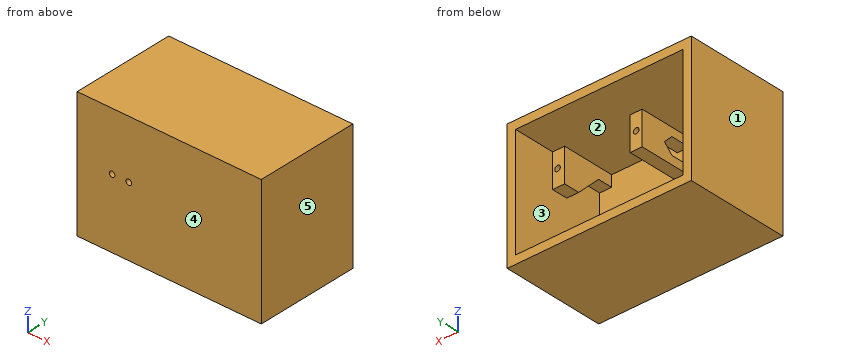
Autodesk Inventor part; units mm, degrees
ref_plane "YZ Plane" through (0, 0, 0) normal (1, 0, 0) x (0, 1, 0)
ref_plane "XZ Plane" through (0, 0, 0) normal (0, 1, 0) x (-1, 0, 0)
ref_plane "XY Plane" through (0, 0, 0) normal (0, 0, 1) x (1, 0, 0)
sketch "스케치1" plane through (0, 0, 0) normal (0, 1, 0) x (-1, 0, 0)
  line L0 (30, 20) -> (-30, 20)
  line L1 (-30, 20) -> (-30, -20)
  line L2 (-30, -20) -> (30, -20)
  line L3 (30, 20) -> (-30, -20) construction
  line L4 (-30, 20) -> (30, -20) construction
  line L5 (30, -20) -> (30, 20)
  line L6 (33, 23) -> (-33, 23)
  line L7 (-33, 23) -> (-33, -23)
  line L8 (-33, -23) -> (33, -23)
  line L9 (33, -23) -> (33, 23)
  point P0 (0, 0)
  dimension "d0" = 60
  dimension "d1" = 40
  dimension "d6" = 3
extrude "돌출1" add sketch "스케치1" against normal blind 3 contours L5 L2 L1 L0 | L9 L8 L7 L6
extrude "돌출2" add sketch "스케치1" along normal blind 34
sketch "스케치2" plane through (0, 0, 0) normal (0, 1, 0) x (1, 0, 0)
  circle A0 centre (-20.5, -2) radius 1
  circle A1 centre (-14.5, -2) radius 1
  line L0 (-30, 20) -> (30, 20)
  line L1 (-30, -20) -> (-30, 20)
  point P0 (0, 0)
  dimension "d11" = 2
  dimension "d12" = 2
  dimension "d13" = 6
  dimension "d14" = 22
  dimension "d15" = 9.5
extrude "돌출3" cut sketch "스케치2" against normal blind 10
sketch "스케치3" plane through (0, 0, 0) normal (0, 1, 0) x (1, 0, 0)
  line L0 (30, -20) -> (-30, -20)
  line L1 (-2.1, -20) -> (2.2, -20)
  line L2 (2.2, -20) -> (2.2, -8)
  line L3 (2.2, -8) -> (-2.1, -8)
  line L4 (-2.1, -8) -> (-2.1, -20)
  line L5 (25.7, -8) -> (30, -8)
  line L6 (30, -8) -> (30, -20)
  line L7 (30, -20) -> (25.7, -20)
  line L8 (25.7, -20) -> (25.7, -8)
  circle A0 centre (0.05, -14) radius 1
  circle A1 centre (28.25, -14) radius 1
  point P0 (0, 0)
  point P1 (0.05, -8)
  point P2 (2.2, -14)
  point P3 (2.2, -20)
  dimension "d18" = 12
  dimension "d19" = 23.5
  dimension "d20" = 32.1
  dimension "d21" = 2
  dimension "d22" = 2
  dimension "d23" = 28.2
extrude "돌출4" add sketch "스케치3" along normal blind 19
sketch "스케치4" plane through (-2.1, 0, 8) normal (-1, 0, 0) x (0, 0, 1)
  line L0 (0, 0) -> (12, 0)
  line L1 (9, 0) -> (3, 0)
  line L2 (3, 0) -> (3, 7)
  line L3 (6, 10) -> (6, 10)
  line L4 (9, 7) -> (9, 0)
  line L5 (3, 7) -> (6, 10)
  line L6 (6, 10) -> (9, 7)
  point P0 (-8, 0)
  point P1 (3, 10)
  point P2 (9, 10)
  point P3 (6, 0)
  point P4 (6, 10)
  point P5 (3, 0)
  dimension "d26" = 6
  dimension "d27" = 10
  dimension "d28" = 3
  dimension "d29" = 3
  dimension "d30" = 3
  dimension "d31" = 3
extrude "돌출5" cut sketch "스케치4" against normal up to surface (4.3 mm away)
sketch "스케치5" plane through (25.7, 0, 8) normal (-1, 0, 0) x (0, 0, 1)
  line L0 (0, 13.3063) -> (8, 5.3063)
  line L1 (8, 5.3063) -> (8, 0)
  line L2 (7, 19) -> (7, 0)
  line L3 (0, 0) -> (-28, 0)
  line L4 (8, 0) -> (0, 0)
  line L5 (0, 0) -> (0, 13.3063)
  point P0 (-8, 0)
  dimension "d34" = 45
  dimension "d35" = 8
extrude "돌출6" cut sketch "스케치5" against normal up to surface (4.3 mm away)
properties part number "전체 하우징"
Build history of the part. All positions in model axes, mm. Face numbers are marked on the shaded views. A direction names the side the tool comes from. Give positions to 0.01 mm unless a question says otherwise; leave off trailing zeros. Loops run counter-clockwise (first coordinate to the right, second up) from the corner with the lowest first, then second, coordinate; pieces in that order, holes last.
Item 1: Slice it at D-D, the plane x = 0.05. List the corners of the cut face in (y, z).
Answers follow:
outline: (-3, -23) - (34, -23) - (34, -20) - (0, -20) - (0, 8) - (19, 8) - (19, 13) - (9, 13) - (7, 11) - (0, 11) - (0, 17) - (7, 17) - (9, 15) - (19, 15) - (19, 20) - (34, 20) - (34, 23) - (-3, 23) - close
Item 2: Flat gauge pins, fed straight in: pin 1 (12 mm diameter, centred on x = -12.5, z = -14.5, fed in from +Y); pin 2 (2 mm diameter, centred on x = 21, z = -16.5, fed in from +Y); pin 3 (1.3 mm diameter, centred on x = 28, z = 14.5, fed in from +Y). Where does each tip first touch, or does it go through?
Answers follow:
pin 1: stops at y = 34
pin 2: stops at y = 0
pin 3: stops at y = 19
Item 3: Which spindle directions (+Z, -Z, +X, -X, +Y, -Y) get a long thin tool onto all of the face, cutting with end or side? Do the marked faces 1 and 2. Say none if no direction does.
Answers follow:
face 1: +Z, -Z, -X, +Y, -Y
face 2: +Y
Item 4: Slice it at A-A, the plane z = 2. List the corners of the cut face in (x, y).
Answers follow:
outline: (-33, -3) - (-21.5, -3) - (-21.5, 0) - (-30, 0) - (-30, 34) - (-33, 34) - close; (-19.5, -3) - (-15.5, -3) - (-15.5, 0) - (-19.5, 0) - close; (-13.5, -3) - (33, -3) - (33, 34) - (30, 34) - (30, 0) - (-13.5, 0) - close
Item 5: Slice it at B-B, the plane x = -14.5. List the corners of the cut face in (y, z).
Answers follow:
outline: (-3, -23) - (34, -23) - (34, -20) - (0, -20) - (0, 1) - (-3, 1) - close; (-3, 3) - (0, 3) - (0, 20) - (34, 20) - (34, 23) - (-3, 23) - close
Item 6: Pull direction X, two halves, no side cores. Call the marked faces 3, 4 and 5: released by +X, released by -X, zero draft, split by the parting line, or undercut.
Answers follow:
face 3: undercut
face 4: zero draft
face 5: released by +X
Item 7: Drill centre lines: line 1 (X direction, y = 13, z = 14); line 2 (Z direction, x = 0.05, y = 16.75); line 3 (X direction, y = 15.5, z = 12). Where is each one in solid material? Low to high.
Answers follow:
line 1: x = -33 to -30, -2.1 to -0.95, 1.05 to 2.2, 25.7 to 27.25, 29.25 to 33
line 2: z = -23 to -20, 8 to 13, 15 to 23
line 3: x = -33 to -30, -2.1 to 2.2, 25.7 to 33
Item 8: Slice it at C-C, the plane y = 20. List the corners of the cut face in (x, z).
Answers follow:
outline: (-33, -23) - (33, -23) - (33, 23) - (-33, 23) - close; hole (-30, -20) - (30, -20) - (30, 20) - (-30, 20) - close
